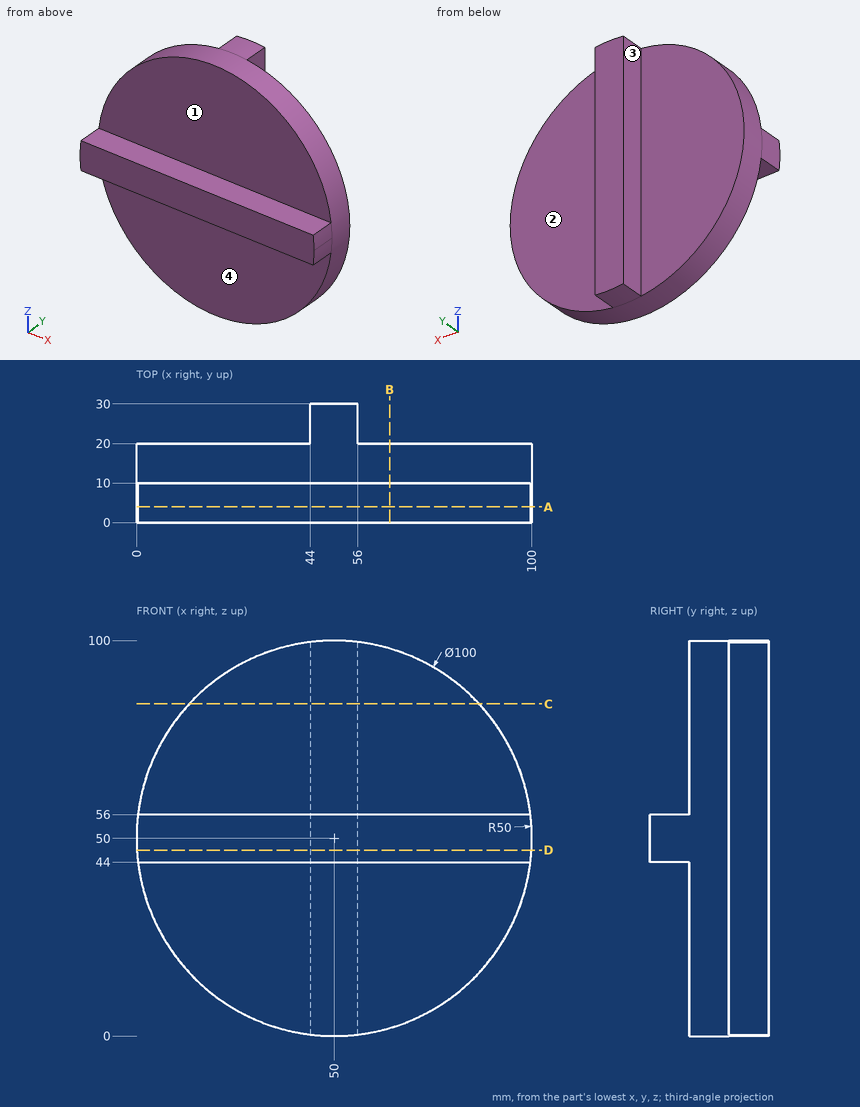
The figure shows three views and two pictorial views of one solid part (mm, origin at its lowest corner). Answer the questions. A direction names the side the tool comes from. Give positions to 0.01 mm unless a question says otherwise; leave off trailing zeros. Write each loop counter-clockwise with the first axis right and the second up, starting at its lowest first coordinate (ties: lowest second). Pieces come first, ordered by that corner, then holes. Notation, with made-up numbers: (-31, 9) -> (-15, 9) arc R34 ccw to (-15, 45) -> close; hole circle Ø5 at (88.5, 64). An arc over 180 degrees is marked (long way). Write each question's results on one line, items separated by ' | '.
1. Find section B-B on x = 64. Determine the outline of the cut face in (y, z), and give its area (3 significant figures).
Data:
outline: (0, 44) -> (10, 44) -> (10, 2) -> (20, 2) -> (20, 98) -> (10, 98) -> (10, 56) -> (0, 56) -> close | area: 1,080 mm^2
2. Find section D-D on z = 47. Determine the outline of the cut face in (x, y).
Data:
outline: (0.09, 0) -> (99.91, 0) -> (99.91, 20) -> (56, 20) -> (56, 30) -> (44, 30) -> (44, 20) -> (0.09, 20) -> close
3. A tool of negligible diameter and unlimited length cuts with its end or side. For the marked faces 1, 2, 3 and 4, from which of +Z, -Z, +X, -X, +Y, -Y can it reach the whole face along a straight path? Write none if from no direction.
Data:
face 1: +Z, +X, -X, -Y | face 2: +Z, -Z, +X, +Y | face 3: +Z, -Z, -X, +Y | face 4: -Z, +X, -X, -Y
4. Find section A-A on y = 4. Determine the outline of the cut face in (x, z).
Data:
outline: (0.36, 44) -> (99.64, 44) arc R50 ccw to (99.64, 56) -> (0.36, 56) arc R50 ccw to start
5. Find section C-C on z = 84. Determine the outline of the cut face in (x, y), and give its area (3 significant figures).
Data:
outline: (13.34, 10) -> (86.66, 10) -> (86.66, 20) -> (56, 20) -> (56, 30) -> (44, 30) -> (44, 20) -> (13.34, 20) -> close | area: 853 mm^2
6. Each of these flat-tipped pins is pushed along its axis until it touches: pin 1 Ø13 at (x, z) = (16, 36.5) entering from +Y; pin 2 Ø22 at (x, z) = (31, 19) entering from -Y; pin 3 Ø1 at (y, z) = (20, 38) entering from -X; pin 4 Ø5 at (x, y) = (34, 24) entering from -Z. Where does it stop, or does it pass through?
Data:
pin 1: y = 20 | pin 2: y = 10 | pin 3: x = 1.34 | pin 4: through
7. Straight lines are drawn through the part: L1, parallel to X at y = 28, z = 66; L2, parallel to Z at x = 50.5, y = 19.25; L3, parallel to Y at x = 6.5, z = 26. For each, find the intervals that lie inside material, in ascending order.
Data:
L1: 44 to 56 | L2: 0 to 100 | L3: 10 to 20
